Geometry check sheet. Reference: drawing and pictorial views, mm from the part's lowest x, y, z. Give positions to 0.01 mm unless a question says otherwise; leave off trailing zeros. Loops run counter-clockwise (first coordinate to the right, second up) from the corner with the lowest first, then second, coordinate; pieces in that order, holes last. Notation, with made-up numbers: (89.5, 34.25) -> (108.5, 34.25) arc R20 cw to (108.5, 60.25) -> close; hole circle Ø1 at (29.25, -36). An arc over 180 degrees is marked (long way). Answer in a Markdown table with one row per item. Add a question column.
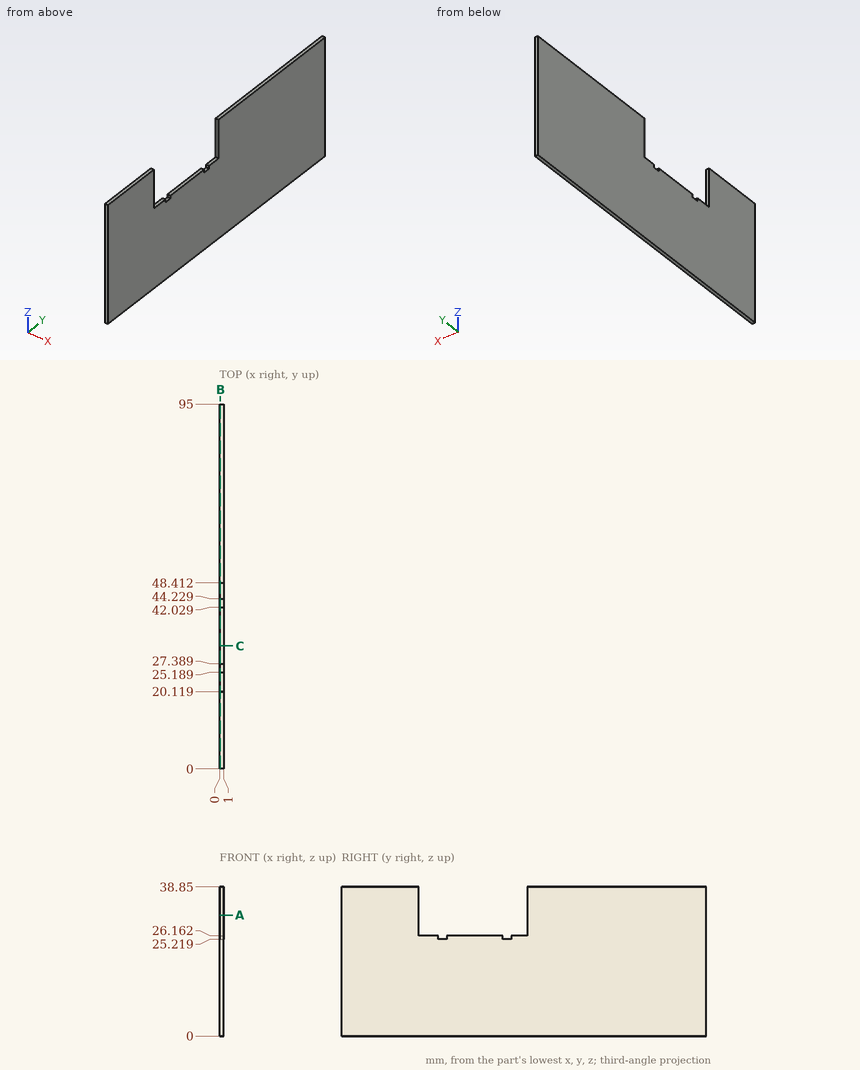
1. Sectioned sample at C-C (y = 32). Enter the section's corners in (x, z).
2. Gauge pin test, flat ends, axial feed: pin 1 Ø5 at (y, z) = (55, 14) entering from -X; pin 2 Ø0.5 at (x, y) = (0.5, 43.5) entering from +Z; pin 3 Ø0.5 at (x, y) = (0.5, 36) entering from +Z. Record the tip position at first contact, or that the pin passes through.
3. Sectioned sample at B-B (x = 0.15). Enter the section's corners in (y, z).
4. Sectioned sample at A-A (z = 31.5). Enter the section's corners in (x, y).
5. Material ranges on L1, parallel to Y at x = 0.85, z = 28; L2, parallel to Z at x = 0.35, y = 21, recorded low to high. Write a range as from..to.
Response:
| question | item | result |
|---|---|---|
| 1 | outline | (0, 0) -> (1, 0) -> (1, 26.16) -> (0, 26.16) -> close |
| 2 | pin 1 | stops at x = 0 |
| 2 | pin 2 | stops at z = 25.22 |
| 2 | pin 3 | stops at z = 26.16 |
| 3 | outline | (0, 0) -> (95, 0) -> (95, 38.85) -> (48.41, 38.85) -> (48.41, 26.16) -> (44.23, 26.16) -> (44.23, 25.22) -> (42.03, 25.22) -> (42.03, 26.16) -> (27.39, 26.16) -> (27.39, 25.22) -> (25.19, 25.22) -> (25.19, 26.16) -> (20.12, 26.16) -> (20.12, 38.85) -> (0, 38.85) -> close |
| 4 | outline | (0, 0) -> (1, 0) -> (1, 20.12) -> (0, 20.12) -> close; (0, 48.41) -> (1, 48.41) -> (1, 95) -> (0, 95) -> close |
| 5 | L1 | y = 0..20.12, 48.41..95 |
| 5 | L2 | z = 0..26.16 |
